```python
from build123d import *

# Parameters (mm, degrees)
F1_DEPTH = 55
F2_R     = 5
F3_T     = -2


# Not quite as in the source:
# - a shell that OpenCascade refuses in one call is made with other operations: the cavity is built on its own and cut out


with BuildPart() as f1:
    # F0 (on Top) → F1 (new body)
    with BuildSketch(Plane.XY):
        with BuildLine():
            Line((-55, -75), (55, -75))
            ThreePointArc((55, -75), (58.5355339059, -73.5355339059), (60, -70))
            Line((60, -70), (60, 70))
            ThreePointArc((60, 70), (58.5355339059, 73.5355339059), (55, 75))
            Line((55, 75), (-55, 75))
            ThreePointArc((-55, 75), (-58.5355339059, 73.5355339059), (-60, 70))
            Line((-60, 70), (-60, -70))
            ThreePointArc((-60, -70), (-58.5355339059, -73.5355339059), (-55, -75))
        make_face()
    extrude(amount=F1_DEPTH)

    # F2
    f2_edges = [f1.edges().sort_by_distance(p)[0] for p in [
        (-60, 0, 55),
        (-60, 0, 0),
    ]]
    fillet(f2_edges, radius=F2_R)

    # F3: a shell. OpenCascade refuses it in one call, so the cavity is built on its own and cut out:
    # the body offset inwards by the wall thickness, plus a prism from it out through each open face.
    f3_core = offset(f1.part, amount=F3_T, mode=Mode.PRIVATE)
    f3_exits = [f3_core.faces().sort_by_distance(p)[0] for p in [
        (0, 0, 53),
    ]]
    add(f3_core, mode=Mode.SUBTRACT)
    extrude(f3_exits, amount=-F3_T, mode=Mode.SUBTRACT)


solid = f1.part
```
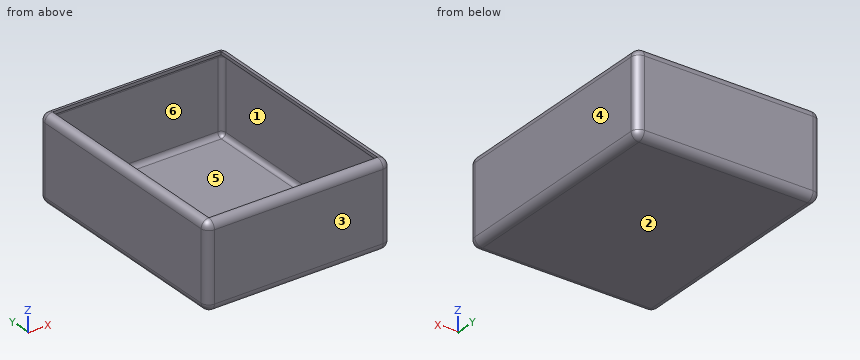
For this review, take the finished solid that the model builds, in its own axes (mm). Face numbers are marked on the shaded views. A direction names the side the tool comes from. Give positions to 0.01 mm unless a question says otherwise; leave off trailing zeros. Write each loop counter-clockwise with the first axis right and the second up, starting at its lowest first coordinate (ties: lowest second). Pieces come first, ordered by that corner, then holes. Notation, with made-up numbers: M -25.75,86.5 L 0.25,86.5 A13 ccw 0.25,99.5 Z; hole C -20.75,89 d7. An arc over 180 degrees is marked long. Answer as CSV lines item,"result".
1. For the marked faces 4, 5 and 6, list the 3-axis set-ups (+Z, -Z, +X, -X, +Y, -Y) from which the entire face can be reached by the end or side of a thin tool; tool diameter is ignored.
Findings:
face 4,"+Z, -Z, +X, +Y, -Y"
face 5,"+Z"
face 6,"none"
2. Draft analysis for pull direction Y (two halves, no side actions). For the marked faces 1, 2 and 3, state which applies: +Y half, -Y half, draft (parallel to the pull), parting line (faces both ways), or undercut.
Findings:
face 1,"undercut"
face 2,"draft"
face 3,"-Y half"
3. Wall thickness on line 1 (Y direction, x = 55, z = 9); line 2 (X direction, y = 64, z = 41.5); line 3 (Z direction, x = -29, y = -65): over which ranges is each line inside the solid? List them lowest first.
Findings:
line 1,"y = -75 to -73, 73 to 75"
line 2,"x = -60 to -58, 58 to 60"
line 3,"z = 0 to 2"
4. Consider section B-B, the plane x = -12.5. Write out the cut boundary in (y, z).
Findings:
outline,"M -75,5 A5 ccw -70,0 L 70,0 A5 ccw 75,5 L 75,50 A5 ccw 70,55 L 70,53 A3 cw 73,50 L 73,5 A3 cw 70,2 L -70,2 A3 cw -73,5 L -73,50 A3 cw -70,53 L -70,55 A5 ccw -75,50 Z"
5. For pin 1 (1.6 mm diameter, centred on y = -22.5, z = 54, fed in from -X); pin 2 (1 mm diameter, centred on x = -44, y = -55.5, fed in from +Z); pin 3 (0.6 mm diameter, centred on y = -31, z = 53.5, fed in from +X), all flat-tipped, find the tip position at first contact; note any pin that passes through.
Findings:
pin 1,"stops at x = -58.84"
pin 2,"stops at z = 2"
pin 3,"stops at x = 58.84"
6. Consider section C-C, the plane y = 9. Write out the cut boundary in (x, z).
Findings:
outline,"M -60,5 A5 ccw -55,0 L 55,0 A5 ccw 60,5 L 60,50 A5 ccw 55,55 L 55,53 A3 cw 58,50 L 58,5 A3 cw 55,2 L -55,2 A3 cw -58,5 L -58,50 A3 cw -55,53 L -55,55 A5 ccw -60,50 Z"
7. Consider section A-A, the plane z = 34. Write out the cut boundary in (x, y).
Findings:
outline,"M -60,-70 A5 ccw -55,-75 L 55,-75 A5 ccw 60,-70 L 60,70 A5 ccw 55,75 L -55,75 A5 ccw -60,70 Z; hole M -58,-70 A3 ccw -55,-73 L 55,-73 A3 ccw 58,-70 L 58,70 A3 ccw 55,73 L -55,73 A3 ccw -58,70 Z"
